Geometry check sheet. Reference: the model listing, model coordinates, mm. Round coordinates to 2 decimals unless told otherwise and drop trailing zeros. Order: outer loops, then holes, each group sorted by start corner. A loop starts at its lowest first (then second) coordinate and runs counter-clockwise, first axis right, second up. Notation, with made-up numbers: (48.5, 26.5) -> (75.5, 26.5) arc R12 ccw to (75.5, 30.5) -> close; hole circle Ø7 at (-25.5, 5.5). An arc over 180 degrees is marked (long way). Answer as a JSON object with one key per item and string values. Group by question number.
from build123d import *

# Parameters (mm, degrees)
BOSS_EXTRUDE1_DEPTH              = 1.27
F_10_0_1935_DIAMETER_HOLE2_D     = 4.9149
F_10_0_1935_DIAMETER_HOLE2_DEPTH = 50.8
F_10_0_1935_DIAMETER_HOLE2_TIP   = 1.476584928


with BuildPart() as part:
    # Sketch1 → Boss-Extrude1 (new, symmetric)
    with BuildSketch(Plane(origin=(0, 0, 0), x_dir=(1, 0, 0), z_dir=(0, 1, 0))):
        Polygon((-49.1324746, -114.072394731), (-23.7324746, -114.072394731), (-23.7324746, 0.227605269), (13.838288869, 80.798367536), (107.467367531, 146.358154211), (92.497603039, 166.878050679), (-49.1324746, 67.707602679), align=None)
    extrude(amount=BOSS_EXTRUDE1_DEPTH, both=True)

    # #10 (0.1935) Diameter Hole2
    with Locations(Plane(origin=(0, 1.27, 0), x_dir=(1, 0, 0), z_dir=(0, 1, 0))):
        with Locations((81.413587814, 144.4055404), (60.607125889, 129.836698916), (39.800663964, 115.267857433), (18.994202039, 100.69901595), (-1.812259886, 86.130174466), (-22.618721811, 71.561332983), (-36.4324746, 35.152605269), (-36.4324746, 9.752605269), (-36.4324746, -15.647394731), (-36.4324746, -41.047394731), (-36.4324746, -66.447394731), (-36.4324746, -91.847394731)):
            Hole(F_10_0_1935_DIAMETER_HOLE2_D / 2, depth=F_10_0_1935_DIAMETER_HOLE2_DEPTH)
            with Locations((0, 0, -(F_10_0_1935_DIAMETER_HOLE2_DEPTH + F_10_0_1935_DIAMETER_HOLE2_TIP / 2))):  # 118° drill point
                Cone(0, F_10_0_1935_DIAMETER_HOLE2_D / 2, F_10_0_1935_DIAMETER_HOLE2_TIP, mode=Mode.SUBTRACT)


solid = part.part
Item 1: Mould release check, pull along Z, two halves, no side actions. Record for faces 1 (the flat face through (-5.21, 0.02, -39.95)), 2 (the flat face through (100.09, 0.02, -156.47)), 3 (the cylindrical face through (-38.776, -0.018, 40.309)): pulls with the +Z half, pulls with the -Z half, needs draft (parallel to the pull), parting line crosses it, or undercut.
Item 2: Thickness scan on L1, parallel to X at y = 0.8, z = 89; L2, parallel to X at y = 0.45, z = -146; L3, parallel to Z at x = -22, y = 0.3. Record the ranges inside material, lowest first.
Item 3: Depth check by flat-ended pin: pin 1 Ø5.5 at (x, z) = (-36.43, 91.85) entering from +Y; pin 2 Ø1.5 at (x, y) = (44, -0.5) entering from -Z. Enter the tip coordinate at first touch or a pass-through.
Item 4: Sectioned sample at B-B, the plane z = 73.5. Enter the section's corners in (x, y), then the cut area to 3 significant figures.
Item 5: Sectioned sample at C-C, the plane x = 29. Enter the section's corners in (y, z).
Item 6: Sectioned sample at A-A, the plane y = 0.25. Count the separate pieces of the cut face and the enclosed holes in it, then the cut area to 3 significant figures.
Result:
{
 "1": {"face 1": "pulls with the +Z half", "face 2": "pulls with the -Z half", "face 3": "undercut"},
 "2": {"L1": "x = -49.13 to -23.73", "L2": "x = 62.68 to 79.54, 83.28 to 106.96", "L3": "z = -86.71 to -73.94, -69.18 to -3.94"},
 "3": {"pin 1": "stops at y = 1.27", "pin 2": "stops at z = -133.44"},
 "4": {"outline": "(-49.13, -1.27) -> (-23.73, -1.27) -> (-23.73, 1.27) -> (-49.13, 1.27) -> close", "area": "64.5 mm2"},
 "5": {"outline": "(-1.27, -122.42) -> (1.27, -122.42) -> (1.27, -91.41) -> (-1.27, -91.41) -> close"},
 "6": {"separate pieces": "1", "enclosed holes": "12", "area": "9,470 mm2"}
}
